Part model, mm, in its own coordinate system. A direction names the side the tool comes from. Give positions to 0.01 mm unless a question says otherwise; leave off trailing zeros. Write each loop counter-clockwise with the first axis right and the second up, starting at its lowest first coordinate (ties: lowest second). Pieces come first, ordered by that corner, then holes. Notation, with made-up numbers: (24, 39.5) - (73, 39.5) arc R25 ccw to (73, 76.5) - close; hole circle Ø2 at (-31.75, 24). An arc over 180 degrees is marked (long way). Answer as a JSON object with one key per item and string values. Group by question number.
```python
from build123d import *

# Parameters (mm, degrees)
F0_W      = 42
F0_H      = 42
F1_DEPTH  = 42
F2_W      = 21
F2_H      = 21
F3_DEPTH  = 42
F4_W      = 21
F4_H      = 21
F5_DEPTH  = 21
F6_W      = 21
F6_H      = 21
F7_DEPTH  = 21
F8_W      = 19
F8_H      = 19
F9_DEPTH  = 41
F10_W     = 19
F10_H     = 19
F11_DEPTH = 41
F12_W     = 19
F12_H     = 19
F13_DEPTH = 41
F14_W     = 21
F14_H     = 21
F15_DEPTH = 21
F16_R     = 6
F17_DEPTH = 18


with BuildPart() as f1:
    # F0 (on Top) → F1 (new body)
    with BuildSketch(Plane.XY):
        Rectangle(F0_W, F0_H)
    extrude(amount=F1_DEPTH)

    # F2 (on face) → F3 (cut, through all)
    with BuildSketch(Plane.XY.offset(42)):
        with Locations((-10.5, 10.5)):
            Rectangle(F2_W, F2_H)
    extrude(amount=-F3_DEPTH, mode=Mode.SUBTRACT)

    # F4 (on face) → F5 (cut, through all)
    with BuildSketch(Plane.XZ.offset(21)):
        with Locations((-10.5, 31.5)):
            Rectangle(F4_W, F4_H)
    extrude(amount=-F5_DEPTH, mode=Mode.SUBTRACT)

    # F6 (on face) → F7 (cut, through all)
    with BuildSketch(Plane.YZ.offset(21)):
        with Locations((10.5, 31.5)):
            Rectangle(F6_W, F6_H)
    extrude(amount=-F7_DEPTH, mode=Mode.SUBTRACT)

    # F8 (on face) → F9 (cut)
    with BuildSketch(Plane.XY.offset(42)):
        with Locations((10.5, -10.5)):
            Rectangle(F8_W, F8_H)
    extrude(amount=-F9_DEPTH, mode=Mode.SUBTRACT)

    # F10 (on face) → F11 (cut)
    with BuildSketch(Plane(origin=(-21, 0, 0), x_dir=(0, -1, 0), z_dir=(-1, 0, 0))):
        with Locations((10.5, 10.5)):
            Rectangle(F10_W, F10_H)
    extrude(amount=-F11_DEPTH, mode=Mode.SUBTRACT)

    # F12 (on face) → F13 (cut)
    with BuildSketch(Plane(origin=(0, 21, 0), x_dir=(-1, 0, 0), z_dir=(0, 1, 0))):
        with Locations((-10.5, 10.5)):
            Rectangle(F12_W, F12_H)
    extrude(amount=-F13_DEPTH, mode=Mode.SUBTRACT)

    # F14 (on face) → F15 (join)
    with BuildSketch(Plane(origin=(0, 0, 0), x_dir=(1, 0, 0), z_dir=(0, 0, -1))):
        with Locations((10.5, 10.5)):
            Rectangle(F14_W, F14_H)
    extrude(amount=F15_DEPTH)

    # F16 (on face) → F17 (cut)
    with BuildSketch(Plane(origin=(0, 0, -21), x_dir=(1, 0, 0), z_dir=(0, 0, -1))):
        with Locations((10.5, 10.5)):
            Circle(F16_R)
    extrude(amount=-F17_DEPTH, mode=Mode.SUBTRACT)


solid = f1.part
```
1) Saw through at C-C (y = 14.5). List the corners of the cut face in (x, z).
2) Which spindle directions (+Z, -Z, +X, -X, +Y, -Y) get a long thin tool onto all of the face, cutting with end or side? Do faces 4 (the flat face through (0, -10, -10)), 5 (the cylindrical face through (13.269, -5.177, -12.126)), 6 (the flat face through (20, -4, 17)). Say none if no direction does.
3) Saw through at D-D (y = -10.5). List the corners of the cut face in (x, z).
4) Drill centre lines: line 1 along Z through (x, y) = (-10, -10); line 2 along X through (y, z) = (-10.5, -14.75); line 3 along Y through (x, z) = (17, 30). Where is each one in solid material? Low to high. Write a range as from..to.
5) Drop flat-ended pins along their axis: P1, Ø9.5, axis at x = 10.5, y = -10.5, coming from the +Z side; P2, Ø10, axis at x = -2, z = -12, coming from the +Y side; P3, Ø15, axis at x = -14, y = -10, coming from the -Z side. Give the stop position or say it passes through.
6) Saw through at A-A (x = 10.5). List the corners of the cut face in (y, z).
7) Two-plate mould, pull along Z, no slides. Class faces 1 (the flat face through (11, 10, 21)), 2 (the flat face through (4, -4, 1)), 3 (the flat face through (15, -6, -21)): +Z half, -Z half, draft (parallel to the pull), parting line (faces both ways), or undercut.
8) Saw through at B-B (z = 12.5). List the corners of the cut face in (x, y), and give its area (3 significant figures).
Checks:
{
 "1": {"outline": "(0, 0) - (21, 0) - (21, 21) - (0, 21) - close; hole (1, 1) - (20, 1) - (20, 20) - (1, 20) - close"},
 "2": {"face 4": "-Z, -X, +Y, -Y", "face 5": "-Z", "face 6": "none"},
 "3": {"outline": "(-21, 0) - (0, 0) - (0, -21) - (4.5, -21) - (4.5, -3) - (16.5, -3) - (16.5, -21) - (21, -21) - (21, 42) - (20, 42) - (20, 1) - (-21, 1) - close; (-21, 20) - (1, 20) - (1, 42) - (0, 42) - (0, 21) - (-21, 21) - close"},
 "4": {"line 1": "0..1, 20..21", "line 2": "0..4.5, 16.5..21", "line 3": "-21..-20, -1..0"},
 "5": {"P1": "z = 1", "P2": "y = 0", "P3": "z = 0"},
 "6": {"outline": "(-21, -21) - (-16.5, -21) - (-16.5, -3) - (-4.5, -3) - (-4.5, -21) - (0, -21) - (0, 0) - (21, 0) - (21, 1) - (-20, 1) - (-20, 42) - (-21, 42) - close; (-1, 20) - (21, 20) - (21, 21) - (0, 21) - (0, 42) - (-1, 42) - close"},
 "7": {"face 1": "+Z half", "face 2": "undercut", "face 3": "-Z half"},
 "8": {"outline": "(-21, -21) - (21, -21) - (21, 21) - (20, 21) - (20, -20) - (-21, -20) - close; (-21, -1) - (1, -1) - (1, 21) - (0, 21) - (0, 0) - (-21, 0) - close", "area": "126 mm2"}
}
